Design review of the part built by this model. Coordinates are the model's own, in mm. Face numbers are marked on the shaded views. A direction names the side the tool comes from. Give positions to 0.01 mm unless a question says otherwise; leave off trailing zeros. Loops run counter-clockwise (first coordinate to the right, second up) from the corner with the lowest first, then second, coordinate; pieces in that order, holes last.
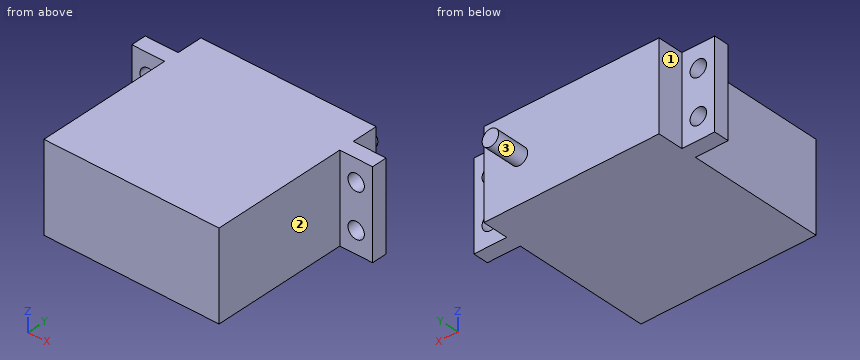
from build123d import *

# Parameters (mm, degrees)
SKETCH1_W                = 40
SKETCH1_H                = 20
BOSS_EXTRUDE1_DEPTH      = 40.5
BOSS_EXTRUDE2_DEPTH      = 7.5
BOSS_EXTRUDE2_DEPTH_BACK = 47.5
SKETCH2_W                = 20
SKETCH2_H                = 3.48
SKETCH3_R                = 1.875
CUT_EXTRUDE1_DEPTH       = 63.075840711
SKETCH4_R                = 1.875
BOSS_EXTRUDE3_DEPTH      = 7.5


with BuildPart() as part:
    # Sketch1 → Boss-Extrude1 (new body)
    with BuildSketch(Plane(origin=(0, 0, 0), x_dir=(1, 0, 0), z_dir=(0, 1, 0))):
        with Locations((20, 10)):
            Rectangle(SKETCH1_W, SKETCH1_H)
    extrude(amount=BOSS_EXTRUDE1_DEPTH)

    # Sketch2 → Boss-Extrude2 (add, two sides: drawn at the far end of the back side and taken through both)
    with BuildSketch(Plane(origin=(40, 0, 0), x_dir=(0, 0, -1), z_dir=(1, 0, 0)).offset(-BOSS_EXTRUDE2_DEPTH_BACK)):
        with Locations((10, 32.86)):
            Rectangle(SKETCH2_W, SKETCH2_H)
    extrude(amount=BOSS_EXTRUDE2_DEPTH + BOSS_EXTRUDE2_DEPTH_BACK)

    # Sketch3 → Cut-Extrude1 (cut, through all)
    with BuildSketch(Plane(origin=(0, 34.6, 0), x_dir=(1, 0, 0), z_dir=(0, 1, 0))):
        with Locations(Location((43.75, 15, 0), (0, 0, 270))):
            Circle(SKETCH3_R)
        with Locations(Location((43.75, 5, 0), (0, 0, 270))):
            Circle(SKETCH3_R)
        with Locations(Location((-3.75, 15, 0), (0, 0, 270))):
            Circle(SKETCH3_R)
        with Locations(Location((-3.75, 5, 0), (0, 0, 270))):
            Circle(SKETCH3_R)
    extrude(amount=-CUT_EXTRUDE1_DEPTH, mode=Mode.SUBTRACT)

    # Sketch4 → Boss-Extrude3 (add)
    with BuildSketch(Plane(origin=(0, 40.5, 0), x_dir=(1, 0, 0), z_dir=(0, 1, 0))):
        with Locations(Location((31.8724, 10, 0), (0, 0, 90))):
            Circle(SKETCH4_R)
    extrude(amount=BOSS_EXTRUDE3_DEPTH)


solid = part.part
Q1. Take a section at C-C (z = -10). Give the boundary of the cut face in (x, y), plus the area to 3 significant figures.
Results:
outline: (-7.5, 31.12) - (0, 31.12) - (0, 0) - (40, 0) - (40, 31.12) - (47.5, 31.12) - (47.5, 34.6) - (40, 34.6) - (40, 40.5) - (33.75, 40.5) - (33.75, 48) - (30, 48) - (30, 40.5) - (0, 40.5) - (0, 34.6) - (-7.5, 34.6) - close
area: 1,700 mm2
Q2. Insertion check: pin 1 (4.5 mm diameter, centred on y = 38, z = -12, fed in from -X); pin 2 (2 mm diameter, centred on x = 33.5, y = 24.5, fed in from +Z); pin 3 (6 mm diameter, centred on x = -5.5, z = -14, fed in from -Y); pin 4 (8 mm diameter, centred on x = -4.5, z = -14.5, fed in from +Y). Each pin has a flat end and moves straight along its axis. Give the tip position at first contact, or say it passes through.
Results:
pin 1: stops at x = 0
pin 2: stops at z = 0
pin 3: stops at y = 31.12
pin 4: stops at y = 34.6
Q3. Take a section at B-B (z = -15). Give the boundary of the cut face in (x, y) (3 decimals), plus the area to 3 significant figures.
Results:
outline: (-7.5, 31.12) - (-5.625, 31.12) - (-5.625, 34.6) - (-7.5, 34.6) - close; (-1.875, 31.12) - (0, 31.12) - (0, 0) - (40, 0) - (40, 31.12) - (41.875, 31.12) - (41.875, 34.6) - (40, 34.6) - (40, 40.5) - (0, 40.5) - (0, 34.6) - (-1.875, 34.6) - close; (45.625, 31.12) - (47.5, 31.12) - (47.5, 34.6) - (45.625, 34.6) - close
area: 1,650 mm2
Q4. Wall thickness on line 1 (X direction, y = 32.45, z = -5) (3 decimals); line 2 (Z direction, x = -3, y = 33); line 3 (X direction, y = 16.5, z = -10.5): over which ranges is each line inside the solid? List them lowest first.
Results:
line 1: x = -7.5 to -5.625, -1.875 to 41.875, 45.625 to 47.5
line 2: z = -20 to -16.72, -13.28 to -6.72, -3.28 to 0
line 3: x = 0 to 40
Q5. Tool access review of the marked faces 1, 2 and 3: name each direction out of +Z, -Z, +X, -X, +Y, -Y from which nothing blocks a thin tool from reaching the whole face with its end or side.
Results:
face 1: +Z, -Z, -X, +Y
face 2: +Z, -Z, +X, -Y
face 3: +Y
Q6. Take a section at D-D (y = 37). Give the boundary of the cut face in (x, z).
Results:
outline: (0, -20) - (40, -20) - (40, 0) - (0, 0) - close
Q7. Take a section at A-A (x = -3.75). Give the boundary of the cut face in (y, z) (3 decimals), plus the area to 3 significant figures.
Results:
outline: (31.12, -20) - (34.6, -20) - (34.6, -16.875) - (31.12, -16.875) - close; (31.12, -13.125) - (34.6, -13.125) - (34.6, -6.875) - (31.12, -6.875) - close; (31.12, -3.125) - (34.6, -3.125) - (34.6, 0) - (31.12, 0) - close
area: 43.5 mm2
